Geometry check sheet. Reference: the model listing, model coordinates, mm. Round coordinates to 2 decimals unless told otherwise and drop trailing zeros. Use a Markdown table: item, result. Add a question column.
Item 1: Material ranges on probe 1 along X at (y, z) = (4, 0); probe 2 along X at (y, z) = (8.25, 1.5); probe 3 along Z at (x, y) = (74, 4), recorded low to high. Write a range as [from, to].
Item 2: Gauge pin test, flat ends, axial feed: pin 1 Ø8 at (y, z) = (6.5, -84.5) entering from -X; pin 2 Ø1 at (x, y) = (-27, 11.5) entering from +Z; pin 3 Ø6 at (x, z) = (121, 0) entering from -Y; pin 4 Ø8 at (x, y) = (41, 8.5) entering from -Z. Record the tip position at first contact, or that the pin passes through.
Item 3: Mould release check, pull along Z, two halves, no side actions. Record for faces 1 (the cylindrical face through (-124.47, 6.9, -27.64)), 2 (the flat face through (86, 14, -76)), 3 (the cylindrical face through (110.55, 6.93, -14.52)): pulls with the +Z half, pulls with the -Z half, needs draft (parallel to the pull), parting line crosses it, or undercut.
from build123d import *

# Parameters (mm, degrees)
SKETCH1_R           = 127.5
SKETCH1_R_2         = 111.5
SKETCH1_R_3         = 2.5
BOSS_EXTRUDE1_DEPTH = 14
CHAMFER1_SIZE       = 2


with BuildPart() as part:
    # Sketch1 → Boss-Extrude1 (new body)
    with BuildSketch(Plane(origin=(0, 0, 0), x_dir=(1, 0, 0), z_dir=(0, 1, 0))):
        with Locations(Location((0, 0, 0), (0, 0, 270))):
            Circle(SKETCH1_R)
        with Locations(Location((0, 0, 0), (0, 0, 270))):
            Circle(SKETCH1_R_2, mode=Mode.SUBTRACT)
        with Locations(Location((0, 121, 0), (0, 0, 270))):
            Circle(SKETCH1_R_3, mode=Mode.SUBTRACT)
        with Locations(Location((121, 0, 0), (0, 0, 270))):
            Circle(SKETCH1_R_3, mode=Mode.SUBTRACT)
        with Locations(Location((0, -121, 0), (0, 0, 270))):
            Circle(SKETCH1_R_3, mode=Mode.SUBTRACT)
        with Locations(Location((-121, 0, 0), (0, 0, 270))):
            Circle(SKETCH1_R_3, mode=Mode.SUBTRACT)
    extrude(amount=BOSS_EXTRUDE1_DEPTH)

    # Chamfer1
    chamfer1_edges = [part.edges().sort_by_distance(p)[0] for p in [
        (0, 0, -111.5),
        (0, 14, -111.5),
    ]]
    chamfer(chamfer1_edges, length=CHAMFER1_SIZE)


solid = part.part
Found:
| question | item | result |
|---|---|---|
| 1 | probe 1 | x = [-127.5, -123.5], [-118.5, -111.5], [111.5, 118.5], [123.5, 127.5] |
| 1 | probe 2 | x = [-127.49, -123], [-119, -111.49], [111.49, 119], [123, 127.49] |
| 1 | probe 3 | z = [-103.83, -83.4], [83.4, 103.83] |
| 2 | pin 1 | stops at x = -98.87 |
| 2 | pin 2 | stops at z = 124.72 |
| 2 | pin 3 | stops at y = 0 |
| 2 | pin 4 | stops at z = -122.01 |
| 3 | face 1 | parting line crosses it |
| 3 | face 2 | needs draft |
| 3 | face 3 | undercut |
